For this review, take the finished solid that the model builds, in its own axes (mm). Face numbers are marked on the shaded views. A direction names the side the tool comes from. Give positions to 0.01 mm unless a question says otherwise; leave off trailing zeros. Write each loop counter-clockwise with the first axis right and the second up, starting at its lowest first coordinate (ties: lowest second). Pieces come first, ordered by that corner, then holes. Notation, with made-up numbers: M 45,38 L 85,38 A20 cw 85,72 Z; hole C -12.75,56.25 d11. An arc over 180 degrees is marked long. One line per item, written item: value. Start each with the question number.
Item 1: Clearance check with flat-ended pins moving along their axes: pin 1 Ø2 at (x, y) = (29, 11) entering from +Z; pin 2 Ø10 at (x, y) = (22, 9) entering from -Z; pin 3 Ø4 at (y, z) = (8, 11) entering from +X; pin 4 Ø1.5 at (x, z) = (6.5, 3) entering from -Y. State where each tip first meets the part, or that it passes through.
Item 2: To check wall thickness, follow probe 1 along X at (y, z) = (4, 5). State the ranges of the line that lie inside material, in increasing order.
Item 3: Consider section C-C, the plane x = 24.5. Write out the cut boundary in (y, z), and give its area (3 significant figures).
Item 4: Consider section A-A, the plane y = 7.25. Write out the cut boundary in (x, z), and give its area (3 significant figures).
Item 5: Tool access review of the marked faces 1 and 2: name each direction out of +Z, -Z, +X, -X, +Y, -Y from which nothing blocks a thin tool from reaching the whole face with its end or side.
Item 6: Consider section D-D, the plane z = 18.25. Write out the cut boundary in (x, y), and give its area (3 significant figures).
Item 7: Consider section B-B, the plane y = 15. Write out the cut boundary in (x, z).
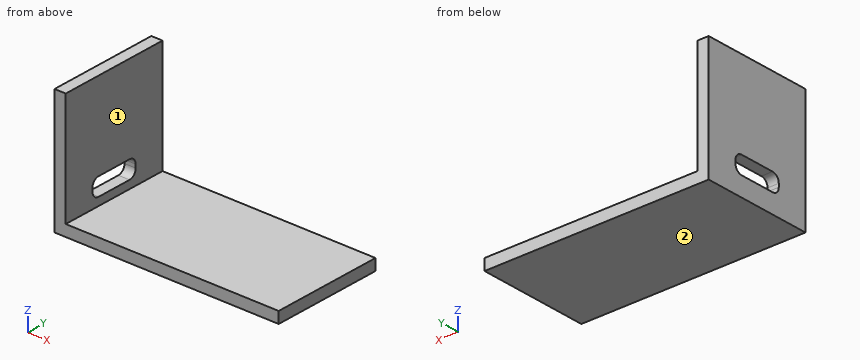
```python
from build123d import *

# Parameters (mm, degrees)
SKETCH_1_W          = 40
SKETCH_1_H          = 20
EXTRUDE_1_DEPTH     = 2
SKETCH_2_W          = 2
SKETCH_2_H          = 20
EXTRUDE_2_DEPTH     = 20
CUT_EXTRUDE_1_DEPTH = 20


with BuildPart() as part:
    # Эскиз1 → Бобышка-Вытянуть1 (new body)
    with BuildSketch(Plane.XY):
        with Locations((20, 10)):
            Rectangle(SKETCH_1_W, SKETCH_1_H)
    extrude(amount=EXTRUDE_1_DEPTH)

    # Эскиз2 → Бобышка-Вытянуть2 (add)
    with BuildSketch(Plane.XY.offset(2)):
        with Locations((1, 10)):
            Rectangle(SKETCH_2_W, SKETCH_2_H)
    extrude(amount=EXTRUDE_2_DEPTH)

    # Эскиз5 → Вырез-Вытянуть1 (cut)
    with BuildSketch(Plane(origin=(2, 0, 0), x_dir=(0, 0, -1), z_dir=(1, 0, 0))):
        with BuildLine():
            Line((-4.699152759, 14.454165244), (-5.299152759, 14.454165244))
            ThreePointArc((-5.299152759, 14.454165244), (-6.204249439, 14.079261924), (-6.579152759, 13.174165244))
            Line((-6.579152759, 13.174165244), (-6.579152759, 6.794165244))
            ThreePointArc((-6.579152759, 6.794165244), (-6.204249439, 5.889068564), (-5.299152759, 5.514165244))
            Line((-5.299152759, 5.514165244), (-4.699152759, 5.514165244))
            ThreePointArc((-4.699152759, 5.514165244), (-3.794056079, 5.889068564), (-3.419152759, 6.794165244))
            Line((-3.419152759, 6.794165244), (-3.419152759, 13.174165244))
            ThreePointArc((-3.419152759, 13.174165244), (-3.794056079, 14.079261924), (-4.699152759, 14.454165244))
        make_face()
    extrude(amount=-CUT_EXTRUDE_1_DEPTH, mode=Mode.SUBTRACT)


solid = part.part
```
Model answer:
1. pin 1: stops at z = 2
1. pin 2: stops at z = 0
1. pin 3: stops at x = 2
1. pin 4: passes through
2. probe 1: x = 0 to 2
3. outline: M 0,0 L 20,0 L 20,2 L 0,2 Z
3. area: 40.0 mm2
4. outline: M 0,0 L 40,0 L 40,2 L 2,2 L 2,3.42 L 0,3.42 Z; M 0,6.58 L 2,6.58 L 2,22 L 0,22 Z
4. area: 114 mm2
5. face 1: +Z, +X, +Y, -Y
5. face 2: -Z, +X, -X, +Y, -Y
6. outline: M 0,0 L 2,0 L 2,20 L 0,20 Z
6. area: 40.0 mm2
7. outline: M 0,0 L 40,0 L 40,2 L 2,2 L 2,22 L 0,22 Z
